Autodesk Fusion 360 part; units mm, degrees
sketch "Sketch1" plane through (0, 0, 0) normal (1, 0, 0) x (0, 0, -1)
  circle A0 centre (0, 0) radius 8.5
  line L0 (-9.9073, -2.5) -> (12, -2.5)
  circle A1 centre (0, 0) radius 10.5
  line L1 (-7.5, 12) -> (7.5, 12)
  line L2 (-7.5, 12) -> (0, 0)
  line L3 (0, 0) -> (7.5, 12)
  line L4 (-10.5, -0.0107) -> (10.5, -0.0107)
  point P0 (0, 12)
  dimension "d1" = 17
  dimension "d2" = 2.5
  dimension "d5" = 21
  dimension "d6" = 12
  dimension "d7" = 15
extrude "Extrude1" add sketch "Sketch1" along normal blind 6 contours A0 L2 L3 L4 | A0 L2 L3 | A0 A1 L2 L3 | A0 L0 L4
extrude "Extrude2" add sketch "Sketch1" along normal blind 7.8 contours A0 L0 L4
Check sheet for the modelled part. Datum: model origin and axes. Units: mm. A direction names the side the tool comes from. Round coordinates to 2 decimals unless told otherwise and drop trailing zeros. Order: outer loops, then holes, each group sorted by start corner. A loop starts at its lowest first (then second) coordinate and runs counter-clockwise, first axis right, second up. Notation, with made-up numbers: M -23,53.25 L 20,53.25 A17 cw 20,74.25 Z; hole C 16.5,-2.5 d7. An arc over 180 degrees is marked long. Answer in a Markdown table with one row per item.
(1) Section check B-B on x = 1.25. Record the boundary of the cut face in (y, z) (3 decimals).
Findings:
| item | result |
|---|---|
| outline | M -2.5,-8.124 A8.5 ccw 7.208,-4.505 L 8.904,-5.565 A10.5 ccw 8.904,5.565 L 7.208,4.505 A8.5 ccw -2.5,8.124 Z |
(2) Material ranges on line 1 along X through (y, z) = (9.5, 3); line 2 along Y through (x, z) = (4.75, 0.25); line 3 along Y through (x, z) = (3, 5), recorded low to high. Write a range as from..to.
Findings:
| item | result |
|---|---|
| line 1 | x = 0..6 |
| line 2 | y = -2.5..10.5 |
| line 3 | y = -2.5..6.87, 8..9.23 |
(3) Section check D-D on y = 4. Record the boundary of the cut face in (x, z).
Findings:
| item | result |
|---|---|
| outline | M 0,-7.5 L 6,-7.5 L 6,7.5 L 0,7.5 Z |
(4) Section check A-A on z = -4.75. Record the boundary of the cut face in (x, y), plus the area to 3 significant figures.
Findings:
| item | result |
|---|---|
| outline | M 0,-2.5 L 7.8,-2.5 L 7.8,-0.01 L 6,-0.01 L 6,7.05 L 0,7.05 Z; M 0,7.6 L 6,7.6 L 6,9.36 L 0,9.36 Z |
| area | 72.4 mm^2 |
(5) Section check C-C on z = -7.25. Record the boundary of the cut face in (x, y).
Findings:
| item | result |
|---|---|
| outline | M 0,-2.5 L 7.8,-2.5 L 7.8,-0.01 L 6,-0.01 L 6,4.44 L 0,4.44 Z |
(6) Set-up check for faces 1 (the flat face through (4, -2.5, 0)), 2 (the flat face through (3, 8, -5)), 3 (the cylindrical face through (3, 10.5, 0.1)), 4 (the flat face through (7, -0.011, 0)), 5 (the flat face through (3, 8, 5)): record each of +Z, -Z, +X, -X, +Y, -Y from which the full face is reachable in a straight line by a thin tool's end or side.
Findings:
| item | result |
|---|---|
| face 1 | +Z, -Z, +X, -X, -Y |
| face 2 | -Z, +X, -X |
| face 3 | +X, -X, +Y |
| face 4 | +Z, -Z, +X, +Y |
| face 5 | +Z, +X, -X |
(7) Gauge pin test, flat ends, axial feed: pin 1 (0.5 mm diameter, centred on x = 7, z = -3, fed in from +Y); pin 2 (5.5 mm diameter, centred on y = 5.5, z = 2.5, fed in from +X); pin 3 (1.5 mm diameter, centred on x = 6, y = 5.5, fed in from +Z). Record the tip position at first contact, or that the pin passes through.
Findings:
| item | result |
|---|---|
| pin 1 | stops at y = -0.01 |
| pin 2 | stops at x = 6 |
| pin 3 | stops at z = 7.05 |
